from build123d import *

# Parameters (mm, degrees)
F1_DEPTH = 10
F2_R     = 5
F4_D     = 6
F6_D     = 12
F7_R     = 1


with BuildPart() as f1:
    # F0 (on Top) → F1 (new body)
    with BuildSketch(Plane.XY):
        with BuildLine():
            Line((20, 30), (-20, 30))
            Line((-20, 30), (-20, 10))
            Line((-20, 10), (-30, 10))
            ThreePointArc((-30, 10), (-40, 0), (-30, -10))
            Line((-30, -10), (-20, -10))
            Line((-20, -10), (-20, -30))
            Line((-20, -30), (20, -30))
            Line((20, -30), (20, 30))
        make_face()
    extrude(amount=F1_DEPTH)

    # F2
    f2_edges = [f1.edges().sort_by_distance(p)[0] for p in [
        (-20, 30, 5),
        (-20, -30, 5),
        (20, -30, 5),
        (20, 30, 5),
        (-20, -10, 5),
        (-20, 10, 5),
    ]]
    fillet(f2_edges, radius=F2_R)

    # F4 (through all)
    with Locations(Plane.XY.offset(10)):
        with Locations((-10, 20), (10, 20), (10, -20), (-10, -20)):
            Hole(F4_D / 2)

    # F6 (through all)
    with Locations(Plane.XY.offset(10)):
        with Locations((-30, 0)):
            Hole(F6_D / 2)

    # F7
    f7_edges = [f1.edges().sort_by_distance(p)[0] for p in [
        (0, 30, 0),
        (0, 30, 10),
    ]]
    fillet(f7_edges, radius=F7_R)


solid = f1.part
Check sheet for the modelled part. Datum: model origin and axes. Units: mm. A direction names the side the tool comes from. Give positions to 0.01 mm unless a question says otherwise; leave off trailing zeros. Loops run counter-clockwise (first coordinate to the right, second up) from the corner with the lowest first, then second, coordinate; pieces in that order, holes last. Notation, with made-up numbers: M 54.5,65.25 L 90.5,65.25 A20 ccw 90.5,79.25 Z; hole C -22,-23.75 d10. An arc over 180 degrees is marked long. Answer as a JSON object with one key per item and string values. Group by question number.
Q1. Cross-section at A-A on y = 0. Record the cut outline in (x, z).
Q2. Cross-section at B-B on x = -10. Record the cut outline in (y, z).
Q3. Go/stop test with flat-tipped pins: P1, Ø1, axis at x = -28, z = 7, coming from the +Y side; P2, Ø2.5, axis at y = -19, z = 6.5, coming from the -X side; P3, Ø1, axis at y = 14, z = 1.5, coming from the -X side; P4, Ø5.5, axis at x = 10, y = -20, coming from the -Z side. Record where each tip stops, or that it passes through.
Q4. Material ranges on line 1 along Y through (x, z) = (-10, 5); line 2 along X through (y, z) = (21.5, 4); line 3 along X through (y, z) = (-23.5, 9), recorded low to high. Write a range as [from, to].
Q5. Cross-section at C-C on y = 20. Record the cut outline in (x, z), then the cut area to 3 significant figures.
Q6. Access from +Z, -Z, +X, -X, +Y, -Y to the whole of each face (thin tool, end or side, straight path). Record for faces 1 (the flat face through (-20, -20, 5)), 2 (the flat face through (0, -30, 5)), 3 (the flat face through (-27, 10, 5)).
Q7. Release check for a two-part mould opening along X. For faces 4 (the cylindrical face through (-11.384, -22.662, 4.93)), 5 (the cylindrical face through (-40, 0, 5)), 6 (the flat face through (-4, 0, 10)) record: released by +X, released by -X, zero draft, split by the parting line, or undercut.
Q8. Cross-section at D-D on z = 4. Record the cut outline in (x, y), then the cut area to 3 significant figures.
Evaluation:
{
 "1": {"outline": "M -40,1 A1 ccw -39,0 L -36,0 L -36,10 L -39,10 A1 ccw -40,9 Z; M -24,0 L 19,0 A1 ccw 20,1 L 20,9 A1 ccw 19,10 L -24,10 Z"},
 "2": {"outline": "M -30,1 A1 ccw -29,0 L -23,0 L -23,10 L -29,10 A1 ccw -30,9 Z; M -17,0 L 17,0 L 17,10 L -17,10 Z; M 23,0 L 29,0 A1 ccw 30,1 L 30,9 A1 ccw 29,10 L 23,10 Z"},
 "3": {"P1": "stops at y = 10", "P2": "stops at x = -20", "P3": "stops at x = -20.23", "P4": "passes through"},
 "4": {"line 1": "y = [-30, -23], [-17, 17], [23, 30]", "line 2": "x = [-20, -12.6], [-7.4, 7.4], [12.6, 20]", "line 3": "x = [-20, 20]"},
 "5": {"outline": "M -20,1 A1 ccw -19,0 L -13,0 L -13,10 L -19,10 A1 ccw -20,9 Z; M -7,0 L 7,0 L 7,10 L -7,10 Z; M 13,0 L 19,0 A1 ccw 20,1 L 20,9 A1 ccw 19,10 L 13,10 Z", "area": "279 mm2"},
 "6": {"face 1": "+Z, -Z, -X, -Y", "face 2": "+Z, -Z, +X, -X, -Y", "face 3": "+Z, -Z, -X, +Y"},
 "7": {"face 4": "undercut", "face 5": "released by -X", "face 6": "zero draft"},
 "8": {"outline": "M -30,-10 L -25,-10 A5 cw -20,-15 L -20,-25 A5 ccw -15,-30 L 15,-30 A5 ccw 20,-25 L 20,25 A5 ccw 15,30 L -15,30 A5 ccw -20,25 L -20,15 A5 cw -25,10 L -30,10 A10 ccw Z; hole C -30,0 d12; hole C -10,-20 d6; hole C -10,20 d6; hole C 10,-20 d6; hole C 10,20 d6", "area": "2,520 mm2"}
}
